The listing builds one solid part. Answer for the finished solid, in the listing's coordinates (mm). Face numbers are marked on the shaded views. A direction names the side the tool comes from. Give positions to 0.01 mm unless a question says otherwise; leave off trailing zeros. Write each loop counter-clockwise with the first axis right and the second up, starting at its lowest first coordinate (ties: lowest second). Pieces come first, ordered by that corner, then holes. Notation, with made-up numbers: (89.25, 12.25) -> (141.25, 12.25) arc R28 cw to (141.25, 38.25) -> close; hole circle Ø11 at (-4.75, 63). An arc over 180 degrees is marked (long way). One line per question, with ' | ' between items.
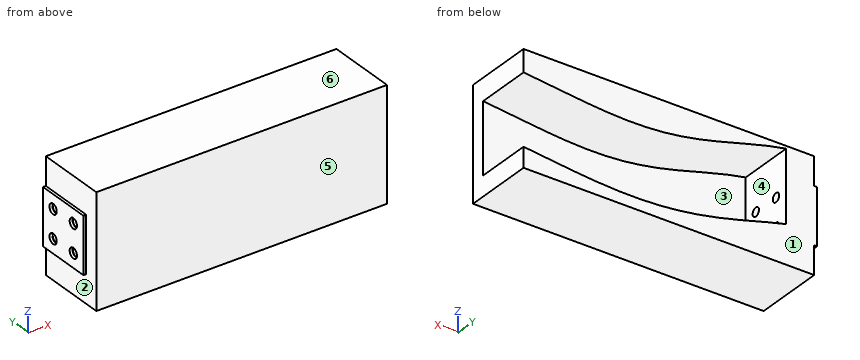
from build123d import *

# Parameters (mm, degrees)
BOSS_EXTRUDE1_DEPTH      = 20
BOSS_EXTRUDE1_DEPTH_BACK = 30
CUT_SWEEP1_START         = -20
CUT_SWEEP1_DEPTH         = 40
SKETCH10_W               = 80
SKETCH10_H               = 50
BOSS_EXTRUDE2_DEPTH      = 20
SKETCH16_W               = 40
SKETCH16_H               = 40
BOSS_EXTRUDE3_DEPTH      = 2
HOLE2_D                  = 6.3
HOLE2_DEPTH              = 22
HOLE2_CBORE_D            = 7.2
HOLE2_CBORE_DEPTH        = 2
SKETCH21_W               = 80
SKETCH21_H               = 50
CUT_EXTRUDE1_DEPTH       = 10


# Read off the part's stored shape, not the designer's step: Cut-Sweep1
with BuildPart() as part:
    # Sketch4 → Boss-Extrude1 (new, two sides: drawn at the far end of the back side and taken through both)
    with BuildSketch(Plane(origin=(0, 0, 0), x_dir=(1, 0, 0), z_dir=(0, 1, 0)).offset(-BOSS_EXTRUDE1_DEPTH_BACK)):
        with BuildLine():
            Line((0, 40.15), (-197, 40.15))
            Line((-197, 40.15), (-197, -12.476031535))
            add(Edge.make_bspline(
                [(-197, -12.476031535), (-157.6, -4.723053252), (-118.2, 15.300441144), (-78.8, 10.012115501), (-39.4, 3.538400001), (0, 0.15)],
                knots=[0.083275556, 0.083275556, 0.083275556, 0.083275556, 0.083275556, 0.083275556, 0.916661414, 0.916661414, 0.916661414, 0.916661414, 0.916661414, 0.916661414], degree=5))
            Line((0, 0.15), (0, 40.15))
        make_face()
        with BuildLine():
            add(Edge.make_bspline(
                [(-197, -12.476031535), (-157.6, -4.723053252), (-118.2, 15.300441144), (-78.8, 10.012115501), (-39.4, 3.538400001), (0, 0.15)],
                knots=[0.083275556, 0.083275556, 0.083275556, 0.083275556, 0.083275556, 0.083275556, 0.916661414, 0.916661414, 0.916661414, 0.916661414, 0.916661414, 0.916661414], degree=5))
            Line((-197, -12.476031535), (-197, -39.85))
            Line((-197, -39.85), (0, -39.85))
            Line((0, -39.85), (0, 0.15))
        make_face()
    extrude(amount=BOSS_EXTRUDE1_DEPTH + BOSS_EXTRUDE1_DEPTH_BACK)

    # Cut-Sweep1 outline → Cut-Sweep1 (cut)
    with BuildSketch(Plane(origin=(0, 0, 0), x_dir=(1, 0, 0), z_dir=(0, 1, 0)).offset(CUT_SWEEP1_START)):
        with BuildLine():
            Line((-197, 12.824466259), (-197, -37.963170516))
            add(Edge.make_bspline(
                [(-197, -37.963170516), (-194.857076562, -37.593469155), (-192.664183232, -37.185688204), (-179.694008515, -34.512721603), (-169.755793181, -31.636726837), (-151.13880736, -26.524050167), (-142.164701345, -24.14456221), (-124.9697813, -20.524403523), (-116.494315107, -19.189461235), (-99.789682062, -17.631352392), (-91.362774073, -17.362930945), (-74.303075644, -17.69764349), (-65.556432968, -18.288800586), (-47.620430646, -19.955725203), (-38.405272349, -21.025808689), (-19.484749512, -23.146908776), (-9.824169485, -24.188286581), (0, -25)],
                knots=[0.098511652, 0.098511652, 0.098511652, 0.098511652, 0.124429736, 0.124429736, 0.248859471, 0.248859471, 0.373289207, 0.373289207, 0.497718942, 0.497718942, 0.622148678, 0.622148678, 0.746578413, 0.746578413, 0.871008149, 0.871008149, 0.995437884, 0.995437884, 0.995437884, 0.995437884], degree=3))
            Line((0, -25), (0, 25))
            add(Edge.make_bspline(
                [(-197, 12.824466259), (-190.953867766, 14.201157707), (-184.535853215, 15.951619244), (-168.3474788, 20.421519224), (-158.563360814, 23.118034358), (-138.248185708, 27.707878723), (-127.968743149, 29.521030359), (-107.155965698, 31.867257342), (-96.8180132, 32.368349134), (-76.327105621, 32.290986848), (-66.286644699, 31.713382561), (-46.616831507, 30.041717947), (-37.012970151, 28.954868939), (-18.255380676, 26.838041894), (-9.05748306, 25.811713394), (0, 25)],
                knots=[0.160277357, 0.160277357, 0.160277357, 0.160277357, 0.248859471, 0.248859471, 0.373289207, 0.373289207, 0.497718942, 0.497718942, 0.622148678, 0.622148678, 0.746578413, 0.746578413, 0.871008149, 0.871008149, 0.995437884, 0.995437884, 0.995437884, 0.995437884], degree=3))
        make_face()
    extrude(amount=CUT_SWEEP1_DEPTH, mode=Mode.SUBTRACT)

    # Sketch10 → Boss-Extrude2 (add)
    with BuildSketch(Plane.ZY.offset(197)):
        with Locations((-0.15, -5)):
            Rectangle(SKETCH10_W, SKETCH10_H)
    extrude(amount=BOSS_EXTRUDE2_DEPTH)

    # Sketch16 → Boss-Extrude3 (add)
    with BuildSketch(Plane.ZY.offset(217)):
        with Locations((-0.15, 0)):
            Rectangle(SKETCH16_W, SKETCH16_H)
    extrude(amount=BOSS_EXTRUDE3_DEPTH)

    # Hole2
    with Locations(Plane.ZY.offset(219)):
        with Locations((-10.15, 10), (9.85, 10), (-10.15, -10), (9.85, -10)):
            CounterBoreHole(HOLE2_D / 2, HOLE2_CBORE_D / 2, HOLE2_CBORE_DEPTH, depth=HOLE2_DEPTH)

    # Sketch21 → Cut-Extrude1 (cut)
    with BuildSketch(Plane(origin=(0, 0, 0), x_dir=(0, 0, -1), z_dir=(1, 0, 0))):
        with Locations((0.15, -5)):
            Rectangle(SKETCH21_W, SKETCH21_H)
    extrude(amount=-CUT_EXTRUDE1_DEPTH, mode=Mode.SUBTRACT)


solid = part.part
Item 1: Consider line 1 (Y direction, x = -218.05, z = -10.15); line 2 (Y direction, x = -218, z = 9); line 3 (X direction, y = -27, z = 35). Determine where each line is inside the solid, lowest interval first. Write a range as [from, to].
Answers below:
line 1: [-20, -13.6], [-6.4, 6.4], [13.6, 20] | line 2: [-20, -13.5], [-6.5, 6.5], [13.5, 20] | line 3: [-217, -10]
Item 2: A tool of negligible diameter and unlimited length cuts with its end or side. For the marked faces 1, 2 and 3, from which of +Z, -Z, +X, -X, +Y, -Y can it reach the whole face along a straight path? Write none if from no direction.
Answers below:
face 1: +Z, -Z, +X, -X, +Y | face 2: -X, -Y | face 3: +Y
Item 3: Flat-ended cylindrical pins translate along their axes: pin 1 (3 mm diameter, centred on x = -133, z = -5.5, fed in from +Y); pin 2 (7 mm diameter, centred on y = -10, z = 9.85, fed in from -X); pin 3 (1 mm diameter, centred on x = -218.5, y = 3.5, fed in from -Z). Find the tip coordinate at first contact, or state that the pin passes through.
Answers below:
pin 1: y = -20 | pin 2: x = -217 | pin 3: z = -20.15
Item 4: Determine the mould class of the marked faces 4, 5 and 6 for opening direction Z: pulls with the +Z half, pulls with the -Z half, needs draft (parallel to the pull), parting line crosses it, or undercut.
Answers below:
face 4: undercut | face 5: needs draft | face 6: pulls with the +Z half
Item 5: Find section A-A (z = -10.15). Write down the section's boundary in (x, y).
Answers below:
outline: (-219, -20) -> (-217, -20) -> (-217, -30) -> (-10, -30) -> (-10, -20) -> (-197, -20) -> (-197, -13.15) -> (-217, -13.15) -> (-217, -13.6) -> (-219, -13.6) -> close; (-219, -6.4) -> (-217, -6.4) -> (-217, -6.85) -> (-197, -6.85) -> (-197, 6.85) -> (-217, 6.85) -> (-217, 6.4) -> (-219, 6.4) -> close; (-219, 13.6) -> (-217, 13.6) -> (-217, 13.15) -> (-197, 13.15) -> (-197, 20) -> (-219, 20) -> close
